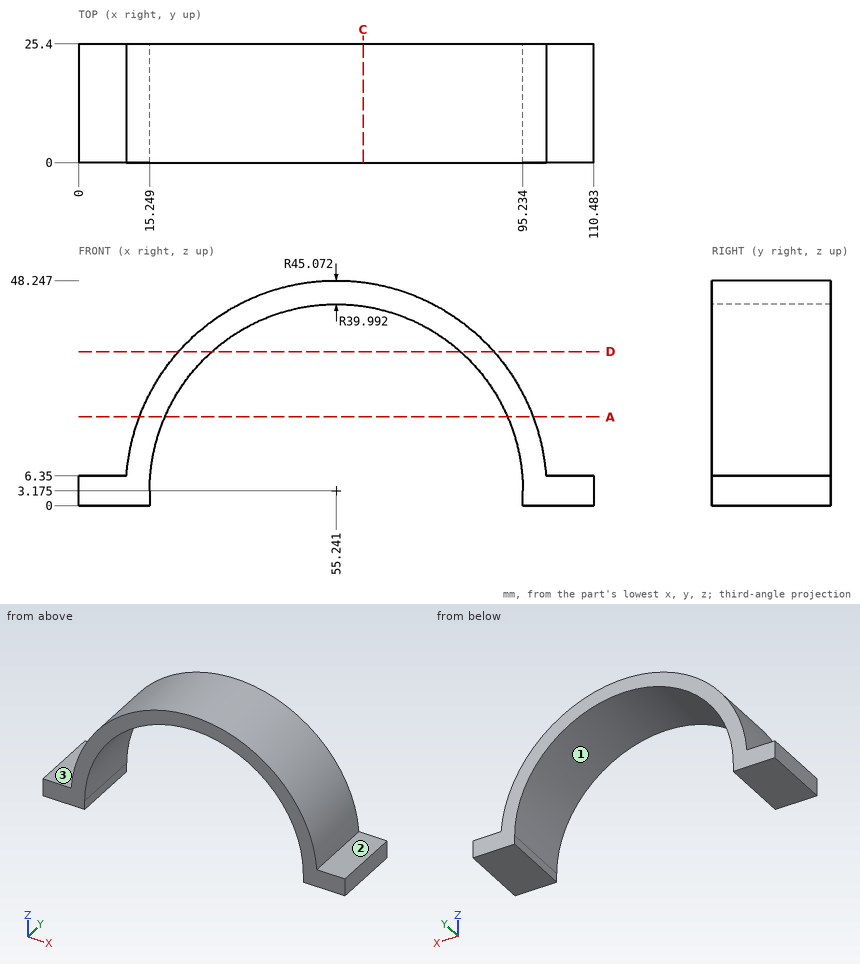
Print and shaded views of the part. All mm, measured from the part's lowest x, y and z. A direction names the side the tool comes from. Coordinates: 2 decimals unless noted, no trailing zeros. Loops run counter-clockwise (first coordinate to the right, second up) from the corner with the lowest first, then second, coordinate; pieces in that order, holes last. Notation, with made-up numbers: M 10,53.5 L 38,53.5 A18 cw 38,57.5 Z; hole C -37,20.25 d8. An arc over 180 degrees is marked long. Use a Markdown table: item, result. Add a question column.
Q1. Which spindle directions (+Z, -Z, +X, -X, +Y, -Y) get a long thin tool onto all of the face, cutting with end or side? Do the marked faces 1, 2 and 3. Say none if no direction does.
Q2. Cut at A-A (z = 19). Write the cut outline in (x, y) (1 decimal), and give its area (3 significant figures).
Q3. Probe L1, parallel to Z at x = 5, y = 17; L2, parallel to X at y = 8.5, z = 26 (1 decimal); L3, parallel to X at y = 1.5, z = 36 (1 decimal). List the from-to ranges inside material, lowest first.
Q4. Cut at D-D (z = 33). Write the cut outline in (x, y) (1 decimal).
Q5. Pin check, flat tips, straight feed: P1, Ø2, axis at y = 22.5, z = 32, coming from the -X side; P2, Ø4, axis at y = 19.5, z = 35.5, coming from the -X side (1 decimal); P3, Ø4, axis at x = 52, y = 21.5, coming from the -Z side. Stop position of each tip, or through.
Q6. Cut at C-C (x = 61). Write the cut outline in (y, z), and give its area (3 significant figures).
Worked out:
| question | item | result |
|---|---|---|
| 1 | face 1 | -Z, +Y, -Y |
| 1 | face 2 | +Z, +X, +Y, -Y |
| 1 | face 3 | +Z, -X, +Y, -Y |
| 2 | outline | M 13,0 L 18.5,0 L 18.5,25.4 L 13,25.4 Z; M 92,0 L 97.4,0 L 97.4,25.4 L 92,25.4 Z |
| 2 | area | 278 mm2 |
| 3 | L1 | z = 0 to 6.35 |
| 3 | L2 | x = 16.4 to 22.4, 88.1 to 94.1 |
| 3 | L3 | x = 24.4 to 32.4, 78.1 to 86.1 |
| 4 | outline | M 21.4,0 L 28.6,0 L 28.6,25.4 L 21.4,25.4 Z; M 81.9,0 L 89,0 L 89,25.4 L 81.9,25.4 Z |
| 5 | P1 | stops at x = 19.78 |
| 5 | P2 | stops at x = 21.9 |
| 5 | P3 | stops at z = 42.82 |
| 6 | outline | M 0,42.75 L 25.4,42.75 L 25.4,47.88 L 0,47.88 Z |
| 6 | area | 130 mm2 |
